```python
from build123d import *

# Parameters (mm, degrees)
F0_R     = 11.1125
F1_DEPTH = 12.7
F2_R     = 3.96875
F3_DEPTH = 53.975
F4_R     = 5.953125
F4_R_2   = 3.96875
F5_DEPTH = 31.75


with BuildPart() as f1:
    # F0 (on Front) → F1 (new body)
    with BuildSketch(Plane.XZ):
        Circle(F0_R)
    extrude(amount=F1_DEPTH)

    # F2 (on Right) → F3 (join)
    with BuildSketch(Plane.YZ):
        with Locations((-7.540625, 0)):
            Circle(F2_R)
    extrude(amount=F3_DEPTH)

    # F4 (on face) → F5 (join)
    with BuildSketch(Plane.YZ.offset(53.975)):
        with Locations((-7.540625, 0)):
            Circle(F4_R)
        with Locations((-7.540625, 0)):
            Circle(F4_R_2, mode=Mode.SUBTRACT)
        with Locations((-7.540625, 0)):
            Circle(F4_R_2)
    extrude(amount=F5_DEPTH)


solid = f1.part
```
Part model, mm, in its own coordinate system. A direction names the side the tool comes from. Round coordinates to 2 decimals unless told otherwise and drop trailing zeros. Order: outer loops, then holes, each group sorted by start corner. A loop starts at its lowest first (then second) coordinate and runs counter-clockwise, first axis right, second up. Notation, with made-up numbers: M 44.5,-10.75 L 73.5,-10.75 A14 ccw 73.5,14.25 Z; hole C 19,81 d5. An arc over 180 degrees is marked long. Answer in a Markdown table with one row per item. Add a question column.
Q1. Mould opens along X. For faces 4 (the face through (85.725, -8, 0)), 5 (the face through (0, 0, 0)), 6 (the face through (31.872, -3.875, -1.52)) say: +X half, -X half, draft (parallel to the pull), parting line (faces both ways), or undercut.
Q2. Cut at B-B on y = -8.5. Give the cut face in (x, z) (1 decimal).
Q3. Cut at D-D on z = 0. Give the cut face in (x, y) (1 decimal), and give its area (3 significant figures).
Q4. Cut at A-A on z = 5. Give the cut face in (x, y) (3 decimals).
Q5. Pin check, flat tips, straight feed: pin 1 (2 mm diameter, centred on x = 47, z = -1.5, fed in from +Y); pin 2 (10 mm diameter, centred on x = 58.5, z = -5, fed in from +Y); pin 3 (1 mm diameter, centred on x = 15, z = 2, fed in from +Y). Stop position of each tip, or through.
Q6. Cut at C-C on x = 21. Give the cut face in (y, z), and give its area (3 significant figures).
Q7. Wall check: L1, parallel to Z at x = 13.5, y = -7.5; L2, parallel to X at y = -5.75, z = -3.75 (3 decimals); L3, parallel to Y at x = 46, z = 1.75. Give the ranges that are in metal, low to high. Write a range as from..to.
Q8. 3-axis set-ups, long thin cutter, end or side, ignore diameter. For faces 1 (the face through (53.975, -6, -4)), 2 (the face through (69.63, -2.04, -2.28)), 3 (the face through (0, -12.7, 0)): which of +Z, -Z, +X, -X, +Y, -Y reach the whole face in a straight line?
Established:
| question | item | result |
|---|---|---|
| 1 | face 4 | +X half |
| 1 | face 5 | draft |
| 1 | face 6 | undercut |
| 2 | outline | M 10.4,-3.9 L 54,-3.9 L 54,-5.9 L 85.7,-5.9 L 85.7,5.9 L 54,5.9 L 54,3.9 L 10.4,3.9 A11.1 ccw long Z |
| 3 | outline | M -11.1,-12.7 L 11.1,-12.7 L 11.1,-11.5 L 54,-11.5 L 54,-13.5 L 85.7,-13.5 L 85.7,-1.6 L 54,-1.6 L 54,-3.6 L 11.1,-3.6 L 11.1,0 L -11.1,0 Z |
| 3 | area | 1,000 mm2 |
| 4 | outline | M -9.924,-12.7 L 9.924,-12.7 L 9.924,0 L -9.924,0 Z; M 53.975,-10.772 L 85.725,-10.772 L 85.725,-4.31 L 53.975,-4.31 Z |
| 5 | pin 1 | stops at y = -3.6 |
| 5 | pin 2 | stops at y = -1.59 |
| 5 | pin 3 | stops at y = -3.87 |
| 6 | outline | C -7.54,0 d7.94 |
| 6 | area | 49.5 mm2 |
| 7 | L1 | z = -3.97..3.97 |
| 7 | L2 | x = -10.461..10.461, 53.975..85.725 |
| 7 | L3 | y = -11.1..-3.98 |
| 8 | face 1 | none |
| 8 | face 2 | +X |
| 8 | face 3 | +Z, -Z, -X, -Y |
